from build123d import *

# Parameters (mm, degrees)
SKETCH1_R           = 4.445
BOSS_EXTRUDE1_DEPTH = 3.937
BOSS_EXTRUDE3_START = -13.208
SKETCH1_5_R         = 4.445
SKETCH1_5_R_2       = 1.2954
SKETCH1_5_W         = 13.97
SKETCH1_5_H         = 24.765
BOSS_EXTRUDE3_DEPTH = 3.937
CUT_EXTRUDE4_DEPTH  = 2.1971
BOSS_EXTRUDE5_DEPTH = 16.4211


with BuildPart() as part:
    # Sketch1 (on Front Plane) → Boss-Extrude1 (new body)
    with BuildSketch(Plane.XY):
        with BuildLine():
            Line((-12.7, 0), (-9.525, 16.51))
            Line((-9.525, 16.51), (9.525, 16.51))
            Line((9.525, 16.51), (12.7, 0))
            Line((12.7, 0), (12.7, -46.99))
            ThreePointArc((12.7, -46.99), (0, -59.69), (-12.7, -46.99))
            Line((-12.7, -46.99), (-12.7, 0))
        make_face()
        Circle(SKETCH1_R, mode=Mode.SUBTRACT)
        with Locations((0, -46.99)):
            Circle(SKETCH1_R, mode=Mode.SUBTRACT)
    extrude(amount=BOSS_EXTRUDE1_DEPTH)

    # Sketch4 → Cut-Extrude4 (cut)
    with BuildSketch(Plane(origin=(0, 0, 0), x_dir=(-1, 0, 0), z_dir=(0, 0, -1))):
        with BuildLine():
            Line((-12.7, 0), (-12.7, -2.669886907))
            Line((-12.7, -2.669886907), (-6.878326735, -4.168384986))
            Line((-6.878326735, -4.168384986), (-2.54, -4.168384986))
            Line((-2.54, -4.168384986), (-2.54, -3.647797281))
            ThreePointArc((-2.54, -3.647797281), (-4.445, 0), (-2.54, 3.647797281))
            Line((-2.54, 3.647797281), (-2.54, 4.168384986))
            Line((-2.54, 4.168384986), (-6.878326735, 4.168384986))
            Line((-6.878326735, 4.168384986), (-12.15982138, 2.808928827))
            Line((-12.15982138, 2.808928827), (-12.7, 0))
        make_face()
        with BuildLine():
            Line((-1.543564577, -4.168384986), (-2.54, -4.168384986))
            Line((-2.54, -4.168384986), (-2.54, -8.89))
            Line((-2.54, -8.89), (2.54, -8.89))
            Line((2.54, -8.89), (2.54, -4.168384986))
            Line((2.54, -4.168384986), (1.543564577, -4.168384986))
            ThreePointArc((1.543564577, -4.168384986), (0, -4.445), (-1.543564577, -4.168384986))
        make_face()
        with BuildLine():
            Line((2.54, -3.647797281), (2.54, -4.168384986))
            Line((2.54, -4.168384986), (6.878326735, -4.168384986))
            Line((6.878326735, -4.168384986), (12.7, -2.669886907))
            Line((12.7, -2.669886907), (12.7, 0))
            Line((12.7, 0), (12.15982138, 2.808928827))
            Line((12.15982138, 2.808928827), (6.878326735, 4.168384986))
            Line((6.878326735, 4.168384986), (2.54, 4.168384986))
            Line((2.54, 4.168384986), (2.54, 3.647797281))
            ThreePointArc((2.54, 3.647797281), (3.940071383, 2.057635172), (4.445, 0))
            ThreePointArc((4.445, 0), (3.940071383, -2.057635172), (2.54, -3.647797281))
        make_face()
        with BuildLine():
            Line((-2.54, 8.89), (-2.54, 4.168384986))
            Line((-2.54, 4.168384986), (-1.543564577, 4.168384986))
            ThreePointArc((-1.543564577, 4.168384986), (0, 4.445), (1.543564577, 4.168384986))
            Line((1.543564577, 4.168384986), (2.54, 4.168384986))
            Line((2.54, 4.168384986), (2.54, 8.89))
            Line((2.54, 8.89), (-2.54, 8.89))
        make_face()
        with BuildLine():
            Line((2.54, 4.168384986), (1.543564577, 4.168384986))
            ThreePointArc((1.543564577, 4.168384986), (2.058307024, 3.939720446), (2.54, 3.647797281))
            Line((2.54, 3.647797281), (2.54, 4.168384986))
        make_face()
        with BuildLine():
            Line((-1.543564577, 4.168384986), (-2.54, 4.168384986))
            Line((-2.54, 4.168384986), (-2.54, 3.647797281))
            ThreePointArc((-2.54, 3.647797281), (-2.058307024, 3.939720446), (-1.543564577, 4.168384986))
        make_face()
        with BuildLine():
            ThreePointArc((2.54, -3.647797281), (2.058307024, -3.939720446), (1.543564577, -4.168384986))
            Line((1.543564577, -4.168384986), (2.54, -4.168384986))
            Line((2.54, -4.168384986), (2.54, -3.647797281))
        make_face()
        with BuildLine():
            Line((-2.54, -3.647797281), (-2.54, -4.168384986))
            Line((-2.54, -4.168384986), (-1.543564577, -4.168384986))
            ThreePointArc((-1.543564577, -4.168384986), (-2.058307024, -3.939720446), (-2.54, -3.647797281))
        make_face()
    extrude(amount=-CUT_EXTRUDE4_DEPTH, mode=Mode.SUBTRACT)



with BuildPart() as body_2:
    # Sketch1<5> → Boss-Extrude3 (new body)
    with BuildSketch(Plane.XY.offset(BOSS_EXTRUDE3_START)):
        with BuildLine():
            Line((-12.7, 0), (-9.525, 16.51))
            Line((-9.525, 16.51), (9.525, 16.51))
            Line((9.525, 16.51), (12.7, 0))
            Line((12.7, 0), (12.7, -46.99))
            ThreePointArc((12.7, -46.99), (0, -59.69), (-12.7, -46.99))
            Line((-12.7, -46.99), (-12.7, 0))
        make_face()
        Circle(SKETCH1_5_R, mode=Mode.SUBTRACT)
        with Locations((0, -10.16)):
            Circle(SKETCH1_5_R_2, mode=Mode.SUBTRACT)
        with Locations((0, -38.1)):
            Circle(SKETCH1_5_R_2, mode=Mode.SUBTRACT)
        with Locations((0, -46.99)):
            Circle(SKETCH1_5_R, mode=Mode.SUBTRACT)
        with Locations((0, -24.13)):
            Rectangle(SKETCH1_5_W, SKETCH1_5_H, mode=Mode.SUBTRACT)
    extrude(amount=-BOSS_EXTRUDE3_DEPTH)


with BuildPart() as part_1:
    add(part.part)

    add(body_2.part)  # Boss-Extrude5 merges body 2
    # Sketch5 → Boss-Extrude5 (add)
    with BuildSketch(Plane(origin=(0, 0, 0), x_dir=(-1, 0, 0), z_dir=(0, 0, -1))):
        Polygon((-9.525, 16.51), (9.525, 16.51), (10.282115385, 12.573), (-10.282115385, 12.573), align=None)
    extrude(amount=BOSS_EXTRUDE5_DEPTH)


solid = part_1.part
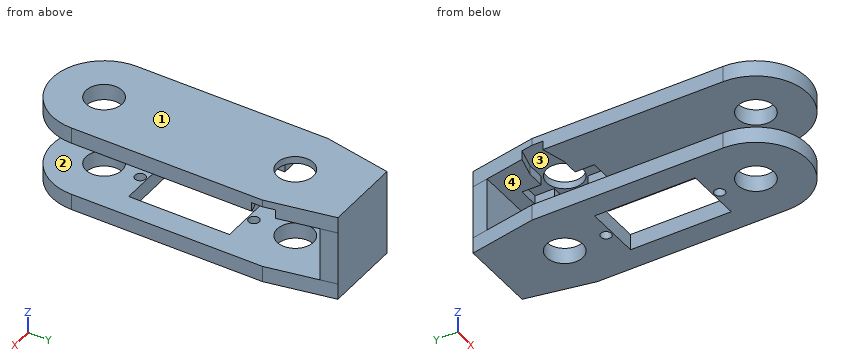
Could you check a few things on this model? Use its own coordinates, in mm. Face numbers are marked on the shaded views. A direction names the side the tool comes from. Give positions to 0.01 mm unless a question says otherwise; leave off trailing zeros. Write each loop counter-clockwise with the first axis right and the second up, starting at its lowest first coordinate (ties: lowest second). Pieces come first, ordered by that corner, then holes. Notation, with made-up numbers: (-18.75, 70) -> (31.25, 70) arc R21 cw to (31.25, 97) -> close; hole circle Ø10 at (-18.5, 51). An arc over 180 degrees is marked (long way). Answer as a JSON object with one key per item and string values.
Q1. Suppose I cut it at B-B on y = -41. Write out the boundary of the cut face in (x, z) (3 decimals).
Taken from the geometry:
{"outline": "(-12.7, -17.145) -> (12.7, -17.145) -> (12.7, -13.208) -> (-12.7, -13.208) -> close; (-12.7, 0) -> (12.7, 0) -> (12.7, 3.937) -> (-12.7, 3.937) -> close"}
Q2. Suppose I cut it at A-A on y = -15. Write out the boundary of the cut face in (x, z) (3 decimals).
Taken from the geometry:
{"outline": "(-12.7, -17.145) -> (-6.985, -17.145) -> (-6.985, -13.208) -> (-12.7, -13.208) -> close; (-12.7, 0) -> (12.7, 0) -> (12.7, 3.937) -> (-12.7, 3.937) -> close; (6.985, -17.145) -> (12.7, -17.145) -> (12.7, -13.208) -> (6.985, -13.208) -> close"}
Q3. Will these pins go through, and if not, where does the flat tip stop? pin 1 Ø4 at (x, z) = (1.5, -6) entering from -Y; pin 2 Ø2.5 at (x, z) = (-5, 1) entering from -Y; pin 3 Ø5 at (y, z) = (-13.5, -3.5) entering from -X; pin 4 Ø8 at (x, y) = (2.5, -16) entering from -Z.
Taken from the geometry:
{"pin 1": "stops at y = 12.57", "pin 2": "stops at y = -59.12", "pin 3": "passes through", "pin 4": "stops at z = 0"}
Q4. Suppose I cut it at D-D on z = -12. Write out the boundary of the cut face in (x, y) (3 decimals), then the cut area to 3 significant figures.
Taken from the geometry:
{"outline": "(-10.282, 12.573) -> (10.282, 12.573) -> (9.525, 16.51) -> (-9.525, 16.51) -> close", "area": "78.0 mm²"}
Q5. Please list where these lines run through material, in increasing order: L1, parallel to Y at x = 0, z = -14.7 (1 decimal); L2, parallel to Z at x = 8.75, y = -45 (3 decimals); L3, parallel to Z at x = 0, y = -6 (3 decimals).
Taken from the geometry:
{"L1": "y = -59.7 to -51.4, -42.5 to -39.4, -36.8 to -36.5, -11.7 to -11.5, -8.9 to -4.4, 4.4 to 16.5", "L2": "z = -17.145 to -13.208, 0 to 3.937", "L3": "z = -17.145 to -13.208, 2.197 to 3.937"}
Q6. Which directions (+Z, -Z, +X, -X, +Y, -Y) give clear straight access to the entire face, cutting with the end or side of a thin tool? Please do the marked faces 1 and 2.
Taken from the geometry:
{"face 1": "+Z, +X, -X, +Y, -Y", "face 2": "+X, -X, -Y"}
Q7. Suppose I cut it at C-C on x = 0. Count the separate pieces of the cut face and the enclosed holes in it, then the cut area to 3 significant figures.
Taken from the geometry:
{"separate pieces": "8", "enclosed holes": "0", "area": "375 mm²"}
Q8. We'd pull the mould along X, two halves only. Please class the marked faces 3 and 4: released by +X, released by -X, zero draft, split by the parting line, or undercut.
Taken from the geometry:
{"face 3": "undercut", "face 4": "zero draft"}
